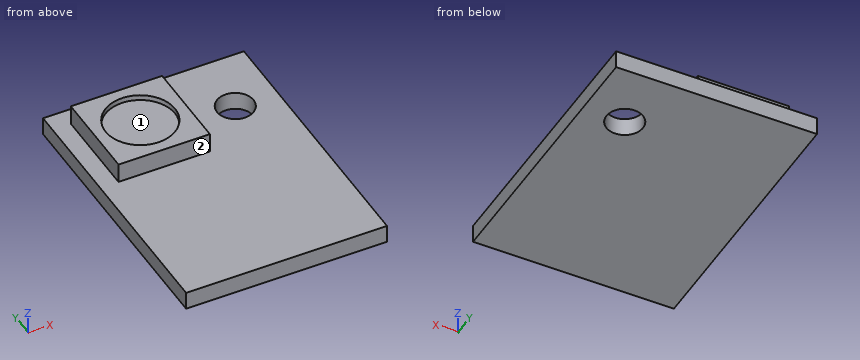
```python
from build123d import *

# Parameters (mm, degrees)
SKETCH_W     = 11
SKETCH_H     = 15
SKETCH_R     = 1
PAD_DEPTH    = 1
SKETCH001_W  = 5
SKETCH001_H  = 5
PAD001_DEPTH = 1.1
SKETCH002_R  = 1.9
POCKET_DEPTH = 0.3


with BuildPart() as part:
    # Sketch → Pad (new body)
    with BuildSketch(Plane.XY):
        with Locations((5.5, 7.5)):
            Rectangle(SKETCH_W, SKETCH_H)
        with Locations((8.7, 11.5)):
            Circle(SKETCH_R, mode=Mode.SUBTRACT)
    extrude(amount=PAD_DEPTH)

    # Sketch001 (on Face7 of Pad) → Pad001 (join)
    with BuildSketch(Plane.XY.offset(1)):
        with Locations((3.5, 11.5)):
            Rectangle(SKETCH001_W, SKETCH001_H)
    extrude(amount=PAD001_DEPTH)

    # Sketch002 (on Face12 of Pad001) → Pocket (cut)
    with BuildSketch(Plane.XY.offset(2.1)):
        with Locations((3.5, 11.5)):
            Circle(SKETCH002_R)
    extrude(amount=-POCKET_DEPTH, mode=Mode.SUBTRACT)


solid = part.part
```
Here's how the part is built. I have some questions about the finished solid (model axes, mm). Face numbers are marked on the shaded views. Give positions to 0.01 mm unless a question says otherwise; leave off trailing zeros. Order: outer loops, then holes, each group sorted by start corner. A loop starts at its lowest first (then second) coordinate and runs counter-clockwise, first axis right, second up. Notation, with made-up numbers: (22.25, -35.75) - (53.25, -35.75) arc R10 cw to (53.25, -28.75) - close; hole circle Ø10 at (37.25, -34). An arc over 180 degrees is marked (long way). Answer as a JSON object with one key per item and string values. Group by question number.
Item 1: If we section it at D-D on z = 0.35: Please give me the cut outline in (x, y), and give its area (3 significant figures).
Item 2: If we section it at B-B on y = 11.5: Please give me the cut outline in (x, z).
Item 3: For P1, Ø1.9, axis at x = 3, y = 10.5, coming from the +Z side; P2, Ø0.9, axis at x = 4.5, z = 1.5, coming from the +Y side; P3, Ø2.5, axis at x = 8.7, y = 11.5, coming from the +Z side; P4, Ø0.9, axis at y = 12, z = 1.5, coming from the +X side, each with a flat end and sliding along its axis, tell me the tip position at first contact or that it passes through.
Item 4: Please list where these lines run through material, in increasing order: probe 1 along Y at (x, z) = (8.7, 0.2); probe 2 along Y at (x, z) = (3.5, 2); probe 3 along Z at (x, y) = (1.5, 1.25).
Item 5: If we mould it in two halves opening along X, with no side actions, what happens to the marked faces 1 and 2? For each: pulls with the +X half, pulls with the -X half, needs draft (parallel to the pull), parting line crosses it, or undercut.
Item 6: If we section it at C-C on x = 3.5: Please give me the cut outline in (y, z).
Item 7: If we section it at A-A on x = 8.7: Please give me the cut outline in (y, z), and give its area (3 significant figures).
Result set:
{
 "1": {"outline": "(0, 0) - (11, 0) - (11, 15) - (0, 15) - close; hole circle Ø2 at (8.7, 11.5)", "area": "162 mm²"},
 "2": {"outline": "(0, 0) - (7.7, 0) - (7.7, 1) - (6, 1) - (6, 2.1) - (5.4, 2.1) - (5.4, 1.8) - (1.6, 1.8) - (1.6, 2.1) - (1, 2.1) - (1, 1) - (0, 1) - close; (9.7, 0) - (11, 0) - (11, 1) - (9.7, 1) - close"},
 "3": {"P1": "z = 2.1", "P2": "y = 14", "P3": "z = 1", "P4": "x = 6"},
 "4": {"probe 1": "0 to 10.5, 12.5 to 15", "probe 2": "9 to 9.6, 13.4 to 14", "probe 3": "0 to 1"},
 "5": {"face 1": "undercut", "face 2": "needs draft"},
 "6": {"outline": "(0, 0) - (15, 0) - (15, 1) - (14, 1) - (14, 2.1) - (13.4, 2.1) - (13.4, 1.8) - (9.6, 1.8) - (9.6, 2.1) - (9, 2.1) - (9, 1) - (0, 1) - close"},
 "7": {"outline": "(0, 0) - (10.5, 0) - (10.5, 1) - (0, 1) - close; (12.5, 0) - (15, 0) - (15, 1) - (12.5, 1) - close", "area": "13.0 mm²"}
}
